Part model, mm, in its own coordinate system. Face numbers are marked on the shaded views. A direction names the side the tool comes from. Give positions to 0.01 mm unless a question says otherwise; leave off trailing zeros. Order: outer loops, then holes, each group sorted by start corner. A loop starts at its lowest first (then second) coordinate and runs counter-clockwise, first axis right, second up. Notation, with made-up numbers: (9, -28.5) - (18, -28.5) arc R13 cw to (18, -21.5) - close; hole circle Ø2 at (30, 39). An arc over 180 degrees is marked (long way). One line per item, written item: value.
```python
from build123d import *

# Parameters (mm, degrees)
F0_W     = 43
F0_H     = 20
F1_DEPTH = 10
F2_D     = 6
F3_W     = 23
F3_H     = 5
F4_DEPTH = 10


with BuildPart() as f1:
    # F0 (on Top) → F1 (new body)
    with BuildSketch(Plane.XY):
        Rectangle(F0_W, F0_H)
    extrude(amount=F1_DEPTH)

    # F2 (through all)
    with Locations(Plane(origin=(0, 0, 0), x_dir=(1, 0, 0), z_dir=(0, 0, -1))):
        with Locations((13.5, 0)):
            Hole(F2_D / 2)

    # F3 (on face) → F4 (cut)
    with BuildSketch(Plane(origin=(0, 0, 0), x_dir=(1, 0, 0), z_dir=(0, 0, -1))):
        with Locations((-10, 7.5)):
            Rectangle(F3_W, F3_H)
    extrude(amount=-F4_DEPTH, mode=Mode.SUBTRACT)


solid = f1.part
```
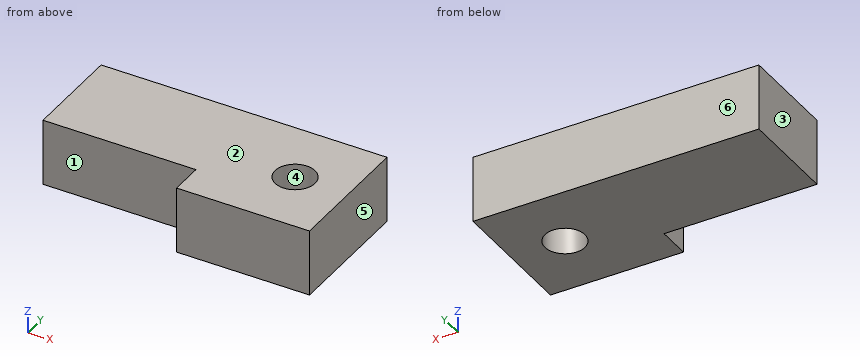
1) Cut at C-C, the plane z = 2. Give the cut face in (x, y).
Outcome:
outline: (-21.5, -5) - (1.5, -5) - (1.5, -10) - (21.5, -10) - (21.5, 10) - (-21.5, 10) - close; hole circle Ø6 at (13.5, 0)
2) Which spindle directions (+Z, -Z, +X, -X, +Y, -Y) get a long thin tool onto all of the face, cutting with end or side? Do the marked faces 1 and 2. Say none if no direction does.
Outcome:
face 1: +Z, -Z, -X, -Y
face 2: +Z, +X, -X, +Y, -Y
3) Cut at D-D, the plane y = -8.25. Give the cut face in (x, z), then the cut area to 3 significant figures.
Outcome:
outline: (1.5, 0) - (21.5, 0) - (21.5, 10) - (1.5, 10) - close
area: 200 mm^2
4) Cut at B-B, the plane y = 0. Give the cut face in (x, z).
Outcome:
outline: (-21.5, 0) - (10.5, 0) - (10.5, 10) - (-21.5, 10) - close; (16.5, 0) - (21.5, 0) - (21.5, 10) - (16.5, 10) - close
5) Drill centre lines: line 1 along Y through (x, z) = (13.5, 4); line 2 along Y through (x, z) = (-15.5, 4.75); line 3 along X through (y, z) = (-7.25, 8.25). Where is each one in solid material? Low to high. Write a range as from..to.
Outcome:
line 1: y = -10..-3, 3..10
line 2: y = -5..10
line 3: x = 1.5..21.5
6) Mould opens along X. For the marked faces 3, 4, 5 and 6 say: released by +X, released by -X, zero draft, split by the parting line, or undercut.
Outcome:
face 3: released by -X
face 4: undercut
face 5: released by +X
face 6: zero draft
7) Pin check, flat tips, straight feed: pin 1 (1 mm diameter, centred on x = -6, z = 4, fed in from -Y); pin 2 (3.5 mm diameter, centred on x = 13.5, y = 0, fed in from -Z); pin 3 (5.5 mm diameter, centred on y = -8, z = 2.5, fed in from -X). Stop position of each tip, or through.
Outcome:
pin 1: stops at y = -5
pin 2: passes through
pin 3: stops at x = 1.5
8) Cut at A-A, the plane x = 13.5. Give the cut face in (y, z), then the cut area to 3 significant figures.
Outcome:
outline: (-10, 0) - (-3, 0) - (-3, 10) - (-10, 10) - close; (3, 0) - (10, 0) - (10, 10) - (3, 10) - close
area: 140 mm^2
